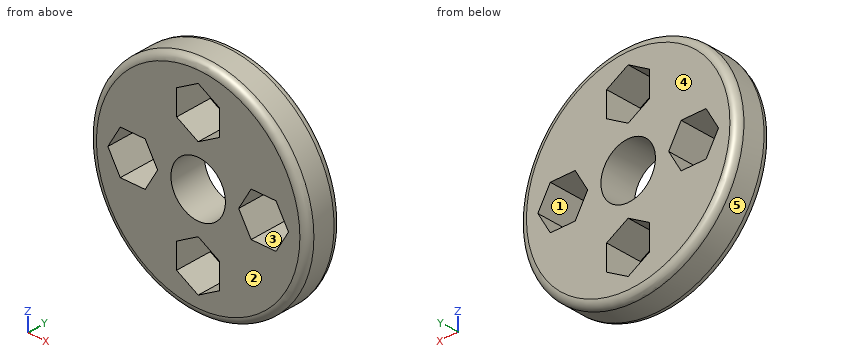
from build123d import *

# Parameters (mm, degrees)
SKETCH1_R           = 30
BOSS_EXTRUDE1_DEPTH = 10
SKETCH2_R           = 7.5
CUT_EXTRUDE1_DEPTH  = 11
FILLET1_R           = 2
CUT_EXTRUDE2_DEPTH  = 11
CIRPATTERN1_COUNT   = 4


with BuildPart() as part:
    # Sketch1 → Boss-Extrude1 (new body)
    with BuildSketch(Plane(origin=(0, 0, 0), x_dir=(1, 0, 0), z_dir=(0, 1, 0))):
        Circle(SKETCH1_R)
    extrude(amount=BOSS_EXTRUDE1_DEPTH)

    # Sketch2 → Cut-Extrude1 (cut, through all)
    with BuildSketch(Plane(origin=(0, 10, 0), x_dir=(1, 0, 0), z_dir=(0, 1, 0))):
        Circle(SKETCH2_R)
    extrude(amount=-CUT_EXTRUDE1_DEPTH, mode=Mode.SUBTRACT)

    # Fillet1
    fillet1_edges = [part.edges().sort_by_distance(p)[0] for p in [
        (-30, 0, 0),
        (-30, 10, 0),
    ]]
    fillet(fillet1_edges, radius=FILLET1_R)

    # Sketch3 → Cut-Extrude2 (cut, through all)
    with BuildSketch(Plane(origin=(0, 10, 0), x_dir=(1, 0, 0), z_dir=(0, 1, 0))):
        Polygon((0, 11.151208395), (5.936478896, 14.578636083), (5.936478896, 21.43349146), (0, 24.860919148), (-5.936478896, 21.43349146), (-5.936478896, 14.578636083), align=None)
    cut_extrude2 = extrude(amount=-CUT_EXTRUDE2_DEPTH, mode=Mode.SUBTRACT)

    # CirPattern1: Cut-Extrude2 ×4 about axis
    cirpattern1_axis = Axis((0, 0, 0), (0, 1, 0))
    for i in range(1, CIRPATTERN1_COUNT):
        add(cut_extrude2.rotate(cirpattern1_axis, i * 360 / CIRPATTERN1_COUNT), mode=Mode.SUBTRACT)


solid = part.part
Can you work these out from the model? Positions are in its coordinate system, mm. Face numbers are marked on the shaded views. A direction names the side the tool comes from. Coordinates: 2 decimals unless noted, no trailing zeros. Write each loop counter-clockwise with the first axis right and the second up, starting at its lowest first coordinate (ties: lowest second). Pieces come first, ordered by that corner, then holes. Notation, with made-up numbers: (89.25, -37.5) -> (115.25, -37.5) arc R26 cw to (115.25, -5.5) -> close; hole circle Ø3 at (-12.5, -13). An arc over 180 degrees is marked (long way). Write item = value, one per line.
(1) On a 3-axis mill with a long thin cutter (end or side, diameter ignored), from which of +Z, -Z, +X, -X, +Y, -Y can I reach the whole of each face in a straight line? I mean the marked faces 1 and 2. Say none if no direction works.
Verdict:
face_1 = +Y, -Y
face_2 = +Z, -Z, +X, -X, -Y
(2) Thinking about a two-plate mould opening in Z: for the marked faces 3, 4 and 5, which applies, +Z half, -Z half, draft (parallel to the pull), parting line (faces both ways), or undercut?
Verdict:
face_3 = undercut
face_4 = draft
face_5 = parting line
(3) For pin 1 (5.5 mm diameter, centred on y = 6.5, z = 17, fed in from -X); pin 2 (2 mm diameter, centred on y = 5, z = 17, fed in from +X); pin 3 (3.5 mm diameter, centred on x = 18.5, y = 5.5, fed in from -Z); pin 4 (9 mm diameter, centred on x = 0, z = 0, fed in from +Y), each with a flat end and sliding along its axis, tell me the tip position at first contact or that it passes through.
Verdict:
pin_1 = -26.4
pin_2 = 25.38
pin_3 = -24.89
pin_4 = through
(4) Imagine slicing it at C-C (y = 1). Please give me the cut outline in (x, z).
Verdict:
outline = circle Ø59.46 at (0, 0); hole (-24.86, 0) -> (-21.43, -5.94) -> (-14.58, -5.94) -> (-11.15, 0) -> (-14.58, 5.94) -> (-21.43, 5.94) -> close; hole circle Ø15 at (0, 0); hole (-5.94, -21.43) -> (0, -24.86) -> (5.94, -21.43) -> (5.94, -14.58) -> (0, -11.15) -> (-5.94, -14.58) -> close; hole (-5.94, 14.58) -> (0, 11.15) -> (5.94, 14.58) -> (5.94, 21.43) -> (0, 24.86) -> (-5.94, 21.43) -> close; hole (11.15, 0) -> (14.58, -5.94) -> (21.43, -5.94) -> (24.86, 0) -> (21.43, 5.94) -> (14.58, 5.94) -> close
(5) If I drill on probe 1 along Z at (x, y) = (0, 7.5); probe 2 along X at (y, z) = (2.5, 0.5); probe 3 along X at (y, z) = (6.25, 3), over which ranges is the centre line in solid material (lowest first)?
Verdict:
probe_1 = -30 to -24.86, -11.15 to -7.5, 7.5 to 11.15, 24.86 to 30
probe_2 = -30 to -24.57, -11.44 to -7.48, 7.48 to 11.44, 24.57 to 30
probe_3 = -29.85 to -23.13, -12.88 to -6.87, 6.87 to 12.88, 23.13 to 29.85
(6) Imagine slicing it at A-A (y = 5.5). Please give me the cut outline in (x, z), and give its area (3 significant figures).
Verdict:
outline = circle Ø60 at (0, 0); hole (-24.86, 0) -> (-21.43, -5.94) -> (-14.58, -5.94) -> (-11.15, 0) -> (-14.58, 5.94) -> (-21.43, 5.94) -> close; hole circle Ø15 at (0, 0); hole (-5.94, -21.43) -> (0, -24.86) -> (5.94, -21.43) -> (5.94, -14.58) -> (0, -11.15) -> (-5.94, -14.58) -> close; hole (-5.94, 14.58) -> (0, 11.15) -> (5.94, 14.58) -> (5.94, 21.43) -> (0, 24.86) -> (-5.94, 21.43) -> close; hole (11.15, 0) -> (14.58, -5.94) -> (21.43, -5.94) -> (24.86, 0) -> (21.43, 5.94) -> (14.58, 5.94) -> close
area = 2,160 mm^2
(7) Imagine slicing it at B-B (z = -1.5). State how many separate pieces and enclosed holes the cut face has, and give its area (3 significant figures).
Verdict:
separate_pieces = 4
enclosed_holes = 0
area = 209 mm^2
